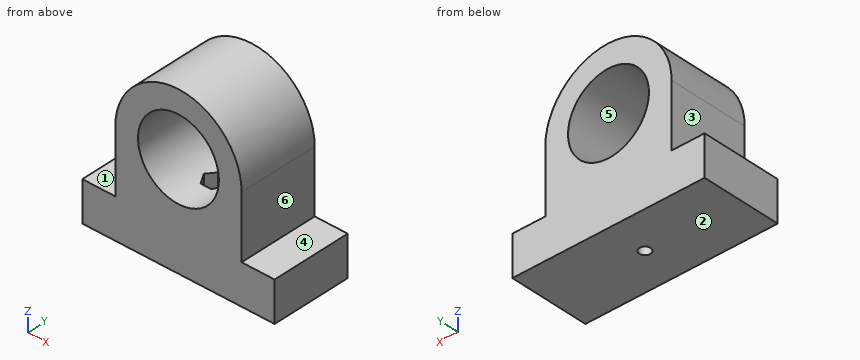
```python
from build123d import *

# Parameters (mm, degrees)
F0_R     = 25.25
F1_DEPTH = 50
F4_D     = 7
F4_DEPTH = 70
F4_TIP   = 2.1030121666
F6_DEPTH = 25


with BuildPart() as f1:
    # F0 (on Front) → F1 (new body)
    with BuildSketch(Plane.XZ):
        with BuildLine():
            ThreePointArc((0, -39.4056375813), (27.8639935507, -27.8639935507), (39.4056375813, 0))
            ThreePointArc((39.4056375813, 0), (0, 39.4056375813), (-39.4056375813, 0))
            ThreePointArc((-39.4056375813, 0), (-27.8639935507, -27.8639935507), (0, -39.4056375813))
        make_face()
        Circle(F0_R, mode=Mode.SUBTRACT)
        with BuildLine():
            ThreePointArc((0, -39.4056375813), (-27.8639935507, -27.8639935507), (-39.4056375813, 0))
            Line((-39.4056375813, 0), (-39.4056375813, -39.4056375813))
            Line((-39.4056375813, -39.4056375813), (0, -39.4056375813))
        make_face()
        Polygon((0, -64.4255876541), (0, -39.4056375813), (-39.4056375813, -39.4056375813), (-60, -39.4056375813), (-60, -64.4255876541), align=None)
        Polygon((39.4056375813, -39.4056375813), (0, -39.4056375813), (0, -64.4255876541), (60, -64.4255876541), (60, -39.4056375813), align=None)
        with BuildLine():
            Line((39.4056375813, -39.4056375813), (39.4056375813, 0))
            ThreePointArc((39.4056375813, 0), (27.8639935507, -27.8639935507), (0, -39.4056375813))
            Line((0, -39.4056375813), (39.4056375813, -39.4056375813))
        make_face()
    extrude(amount=F1_DEPTH)

    # F4
    with Locations(Plane(origin=(0, 0, -64.4255876541), x_dir=(1, 0, 0), z_dir=(0, 0, -1))):
        with Locations((0, 25)):
            Hole(F4_D / 2, depth=F4_DEPTH)
            with Locations((0, 0, -(F4_DEPTH + F4_TIP / 2))):  # 118° drill point
                Cone(0, F4_D / 2, F4_TIP, mode=Mode.SUBTRACT)

    # F5 (on offset) → F6 (cut)
    with BuildSketch(Plane(origin=(0, 0, -39.4255876541), x_dir=(1, 0, 0), z_dir=(0, 0, -1))):
        Polygon((-3.4745540902, 18.9818957821), (3.4745540902, 18.9818957821), (6.9491081805, 25), (3.4745540902, 31.0181042179), (-3.4745540902, 31.0181042179), (-6.9491081805, 25), align=None)
    extrude(amount=-F6_DEPTH, mode=Mode.SUBTRACT)


solid = f1.part
```
Could you check a few things on this model? Use its own coordinates, in mm. Face numbers are marked on the shaded views. A direction names the side the tool comes from. Round coordinates to 2 decimals unless told otherwise and drop trailing zeros. Write each loop counter-clockwise with the first axis right and the second up, starting at its lowest first coordinate (ties: lowest second). Pieces come first, ordered by that corner, then holes. Notation, with made-up numbers: M 77,9 L 99,9 A36 cw 99,43 Z; hole C 5,-37.75 d6. An arc over 180 degrees is marked long. Write each question's results on one line, items separated by ' | '. Start each with the question number.
1. On a 3-axis mill with a long thin cutter (end or side, diameter ignored), from which of +Z, -Z, +X, -X, +Y, -Y can I reach the whole of each face in a straight line? I mean the marked faces 1 and 2. Say none if no direction works.
2. Imagine slicing it at C-C on y = -39. List the corners of the cut face in (x, z) for me, and give its area (3 significant figures).
3. I'm going to push flat-ended pins straight in: pin 1 Ø16.5 at (x, y) = (53.5, -37) entering from +Z; pin 2 Ø12 at (y, z) = (-15, -18) entering from +X; pin 3 Ø2 at (y, z) = (-33, -18.5) entering from -X. Where does each tip first touch, or does it pass through?
4. Imagine slicing it at B-B on z = -36.5. List the corners of the cut face in (x, y) for me, and give its area (3 significant figures).
5. Thinking about a two-plate mould opening in X: for the marked faces 3, 4, 5 and 6, which applies, +X half, -X half, draft (parallel to the pull), parting line (faces both ways), or undercut?
6. Imagine slicing it at D-D on x = 20.5. List the corners of the cut face in (y, z) for me, and give its area (3 significant figures).
7. Imagine slicing it at A-A on x = 0. List the corners of the cut face in (y, z) for me, and give its area (3 significant figures).
8. I need wall thicknesses on L1, parallel to X at y = -25, z = -52.75; L2, parallel to Y at x = 0, z = -53.5; L3, parallel to X at y = -6, z = 3. Which ranges of each line are inside material? Lowest first, please. Write a range as from..to.
Result sheet:
1) face 1: +Z, -X, +Y, -Y | face 2: -Z, +X, -X, +Y, -Y
2) outline: M -60,-64.43 L 60,-64.43 L 60,-39.41 L 39.41,-39.41 L 39.41,0 A39.41 ccw -39.41,0 L -39.41,-39.41 L -60,-39.41 Z; hole C 0,0 d50.5 | area: 6,540 mm^2
3) pin 1: stops at z = -39.41 | pin 2: stops at x = 39.41 | pin 3: stops at x = -39.41
4) outline: M -39.41,-50 L 39.41,-50 L 39.41,0 L -39.41,0 Z; hole M -6.95,-25 L -3.47,-31.02 L 3.47,-31.02 L 6.95,-25 L 3.47,-18.98 L -3.47,-18.98 Z | area: 3,820 mm^2
5) face 3: -X half | face 4: draft | face 5: undercut | face 6: +X half
6) outline: M -50,-64.43 L 0,-64.43 L 0,-14.74 L -50,-14.74 Z; M -50,14.74 L 0,14.74 L 0,33.65 L -50,33.65 Z | area: 3,430 mm^2
7) outline: M -50,-64.43 L -28.5,-64.43 L -28.5,-39.43 L -31.02,-39.43 L -31.02,-25.25 L -50,-25.25 Z; M -50,25.25 L 0,25.25 L 0,39.41 L -50,39.41 Z; M -21.5,-64.43 L 0,-64.43 L 0,-25.25 L -18.98,-25.25 L -18.98,-39.43 L -21.5,-39.43 Z | area: 2,320 mm^2
8) L1: x = -60..-3.5, 3.5..60 | L2: y = -50..-28.5, -21.5..0 | L3: x = -39.29..-25.07, 25.07..39.29
